The listing builds one solid part. Answer for the finished solid, in the listing's coordinates (mm). A direction names the side the tool comes from. Round coordinates to 2 decimals unless told otherwise and drop trailing zeros. Write each loop counter-clockwise with the first axis right and the second up, starting at its lowest first coordinate (ties: lowest second). Pieces come first, ordered by that corner, then holes. Notation, with made-up numbers: M -39,-12 L -7,-12 A33 cw -7,19 Z; hole C 71.5,87 d7. An arc over 180 degrees is marked long. Write each question's results on one line, items separated by ' | '.
from build123d import *

# Parameters (mm, degrees)
SKETCH_1_R          = 42.5
EXTRUDE_1_DEPTH     = 5
SKETCH_2_R          = 5.15
CUT_EXTRUDE_1_DEPTH = 61.311690409
SKETCH_3_R          = 5.15
CUT_EXTRUDE_2_DEPTH = 61.311690409
EXTRUDE_START       = -1
SKETCH_4_R          = 5.15
SKETCH_4_R_2        = 4.15
EXTRUDE_1_2_DEPTH   = 1
CUT_EXTRUDE_3_REACH = 62.312
SKETCH_5_R          = 1.65
CUT_EXTRUDE_4_REACH = 62.312
CUT_EXTRUDE_6_REACH = 62.312
SKETCH_10_R         = 2.15
CUT_EXTRUDE_7_REACH = 62.312
SKETCH_17_W         = 15.112394154
SKETCH_17_H         = 1
EXTRUDE_6_DEPTH     = 5


with BuildPart() as part:
    # 草图1 → Extrude 1 (new body)
    with BuildSketch(Plane.XY):
        Circle(SKETCH_1_R)
    extrude(amount=-EXTRUDE_1_DEPTH)

    # 草图2 → 切除-拉伸1 (cut, through all)
    with BuildSketch(Plane.XY):
        with Locations((-32, 0)):
            Circle(SKETCH_2_R)
        with Locations((-16, 27.712812921)):
            Circle(SKETCH_2_R)
        with Locations((16, 27.712812921)):
            Circle(SKETCH_2_R)
        with Locations((32, 0)):
            Circle(SKETCH_2_R)
        with Locations((16, -27.712812921)):
            Circle(SKETCH_2_R)
        with Locations((-16, -27.712812921)):
            Circle(SKETCH_2_R)
    extrude(amount=-CUT_EXTRUDE_1_DEPTH, mode=Mode.SUBTRACT)

    # 草图3 → 切除-拉伸2 (cut, through all)
    with BuildSketch(Plane.XY):
        Circle(SKETCH_3_R)
    extrude(amount=-CUT_EXTRUDE_2_DEPTH, mode=Mode.SUBTRACT)

    # 草图4 → Extrude 1 2 (add)
    # profile 1 of 6: a face of its own
    with BuildSketch(Plane(origin=(0, 0, -5), x_dir=(-1, 0, 0), z_dir=(0, 0, -1)).offset(EXTRUDE_START)):
        with Locations((-16, 27.712812921)):
            Circle(SKETCH_4_R)
        with Locations((-16, 27.712812921)):
            Circle(SKETCH_4_R_2, mode=Mode.SUBTRACT)
    # profile 2 of 6: a face of its own
    with BuildSketch(Plane(origin=(0, 0, -5), x_dir=(-1, 0, 0), z_dir=(0, 0, -1)).offset(EXTRUDE_START)):
        with Locations((16, 27.712812921)):
            Circle(SKETCH_4_R)
        with Locations((16, 27.712812921)):
            Circle(SKETCH_4_R_2, mode=Mode.SUBTRACT)
    # profile 3 of 6: a face of its own
    with BuildSketch(Plane(origin=(0, 0, -5), x_dir=(-1, 0, 0), z_dir=(0, 0, -1)).offset(EXTRUDE_START)):
        with Locations((32, 0)):
            Circle(SKETCH_4_R)
        with Locations((32, 0)):
            Circle(SKETCH_4_R_2, mode=Mode.SUBTRACT)
    # profile 4 of 6: a face of its own
    with BuildSketch(Plane(origin=(0, 0, -5), x_dir=(-1, 0, 0), z_dir=(0, 0, -1)).offset(EXTRUDE_START)):
        with Locations((16, -27.712812921)):
            Circle(SKETCH_4_R)
        with Locations((16, -27.712812921)):
            Circle(SKETCH_4_R_2, mode=Mode.SUBTRACT)
    # profile 5 of 6: a face of its own
    with BuildSketch(Plane(origin=(0, 0, -5), x_dir=(-1, 0, 0), z_dir=(0, 0, -1)).offset(EXTRUDE_START)):
        with Locations((-16, -27.712812921)):
            Circle(SKETCH_4_R)
        with Locations((-16, -27.712812921)):
            Circle(SKETCH_4_R_2, mode=Mode.SUBTRACT)
    # profile 6 of 6: a face of its own
    with BuildSketch(Plane(origin=(0, 0, -5), x_dir=(-1, 0, 0), z_dir=(0, 0, -1)).offset(EXTRUDE_START)):
        with Locations((-32, 0)):
            Circle(SKETCH_4_R)
        with Locations((-32, 0)):
            Circle(SKETCH_4_R_2, mode=Mode.SUBTRACT)
    extrude(amount=EXTRUDE_1_2_DEPTH)

    # 草图5 → 切除-拉伸3 (cut, up to next)
    with BuildSketch(Plane(origin=(0, 0, -5), x_dir=(-1, 0, 0), z_dir=(0, 0, -1)), mode=Mode.PRIVATE) as cut_extrude_3_sk1:
        with Locations((-16.454482672, 9.5)):
            Circle(SKETCH_5_R)
    cut_extrude_3_tool1 = extrude(cut_extrude_3_sk1.sketch, amount=-CUT_EXTRUDE_3_REACH, mode=Mode.PRIVATE) & part.part
    # 草图5 → 切除-拉伸3 (cut, up to next)
    with BuildSketch(Plane(origin=(0, 0, -5), x_dir=(-1, 0, 0), z_dir=(0, 0, -1)), mode=Mode.PRIVATE) as cut_extrude_3_sk2:
        with Locations((16.454482672, 9.5)):
            Circle(SKETCH_5_R)
    cut_extrude_3_tool2 = extrude(cut_extrude_3_sk2.sketch, amount=-CUT_EXTRUDE_3_REACH, mode=Mode.PRIVATE) & part.part
    # 草图5 → 切除-拉伸3 (cut, up to next)
    with BuildSketch(Plane(origin=(0, 0, -5), x_dir=(-1, 0, 0), z_dir=(0, 0, -1)), mode=Mode.PRIVATE) as cut_extrude_3_sk3:
        with Locations((0, -19)):
            Circle(SKETCH_5_R)
    cut_extrude_3_tool3 = extrude(cut_extrude_3_sk3.sketch, amount=-CUT_EXTRUDE_3_REACH, mode=Mode.PRIVATE) & part.part
    add(cut_extrude_3_tool1.solids().sort_by_distance((16.454483, 9.5, -5))[0], mode=Mode.SUBTRACT)
    add(cut_extrude_3_tool2.solids().sort_by_distance((-16.454483, 9.5, -5))[0], mode=Mode.SUBTRACT)
    add(cut_extrude_3_tool3.solids().sort_by_distance((0, -19, -5))[0], mode=Mode.SUBTRACT)

    # 草图7 → 切除-拉伸4 (cut, up to next)
    with BuildSketch(Plane(origin=(0, 0, -5), x_dir=(-1, 0, 0), z_dir=(0, 0, -1)), mode=Mode.PRIVATE) as cut_extrude_4_sk1:
        with BuildLine():
            Line((-16.495508076, -11.428941916), (-25.155762114, -16.428941916))
            ThreePointArc((-25.155762114, -16.428941916), (-27.40970403, -15.825), (-26.805762114, -13.571058084))
            Line((-26.805762114, -13.571058084), (-18.145508076, -8.571058084))
            ThreePointArc((-18.145508076, -8.571058084), (-15.891566159, -9.175), (-16.495508076, -11.428941916))
        make_face()
    cut_extrude_4_tool1 = extrude(cut_extrude_4_sk1.sketch, amount=-CUT_EXTRUDE_4_REACH, mode=Mode.PRIVATE) & part.part
    add(cut_extrude_4_tool1.solids().sort_by_distance((21.650635, -12.5, -5))[0], mode=Mode.SUBTRACT)

    # 草图10 → 切除-拉伸6 (cut, up to next)
    with BuildSketch(Plane(origin=(0, 0, -5), x_dir=(-1, 0, 0), z_dir=(0, 0, -1)), mode=Mode.PRIVATE) as cut_extrude_6_sk1:
        with Locations((-9.526279442, -5.5)):
            Circle(SKETCH_10_R)
    cut_extrude_6_tool1 = extrude(cut_extrude_6_sk1.sketch, amount=-CUT_EXTRUDE_6_REACH, mode=Mode.PRIVATE) & part.part
    # 草图10 → 切除-拉伸6 (cut, up to next)
    with BuildSketch(Plane(origin=(0, 0, -5), x_dir=(-1, 0, 0), z_dir=(0, 0, -1)), mode=Mode.PRIVATE) as cut_extrude_6_sk2:
        with Locations((0, 11)):
            Circle(SKETCH_10_R)
    cut_extrude_6_tool2 = extrude(cut_extrude_6_sk2.sketch, amount=-CUT_EXTRUDE_6_REACH, mode=Mode.PRIVATE) & part.part
    # 草图10 → 切除-拉伸6 (cut, up to next)
    with BuildSketch(Plane(origin=(0, 0, -5), x_dir=(-1, 0, 0), z_dir=(0, 0, -1)), mode=Mode.PRIVATE) as cut_extrude_6_sk3:
        with Locations((9.526279442, -5.5)):
            Circle(SKETCH_10_R)
    cut_extrude_6_tool3 = extrude(cut_extrude_6_sk3.sketch, amount=-CUT_EXTRUDE_6_REACH, mode=Mode.PRIVATE) & part.part
    add(cut_extrude_6_tool1.solids().sort_by_distance((9.526279, -5.5, -5))[0], mode=Mode.SUBTRACT)
    add(cut_extrude_6_tool2.solids().sort_by_distance((0, 11, -5))[0], mode=Mode.SUBTRACT)
    add(cut_extrude_6_tool3.solids().sort_by_distance((-9.526279, -5.5, -5))[0], mode=Mode.SUBTRACT)

    # 草图11 → 切除-拉伸7 (cut, up to next)
    with BuildSketch(Plane.XY, mode=Mode.PRIVATE) as cut_extrude_7_sk1:
        with BuildLine():
            Line((1.65, 25.457782029), (1.65, 18.457782029))
            ThreePointArc((1.65, 18.457782029), (0, 16.807782029), (-1.65, 18.457782029))
            Line((-1.65, 18.457782029), (-1.65, 25.457782029))
            ThreePointArc((-1.65, 25.457782029), (0, 27.107782029), (1.65, 25.457782029))
        make_face()
    cut_extrude_7_tool1 = extrude(cut_extrude_7_sk1.sketch, amount=-CUT_EXTRUDE_7_REACH, mode=Mode.PRIVATE) & part.part
    add(cut_extrude_7_tool1.solids().sort_by_distance((0, 21.957782, 0))[0], mode=Mode.SUBTRACT)

    # 草图17 → 拉伸-薄壁6 (add)
    with BuildSketch(Plane(origin=(0, 0, -5), x_dir=(-1, 0, 0), z_dir=(0, 0, -1))):
        with Locations((0, 42)):
            Rectangle(SKETCH_17_W, SKETCH_17_H)
    extrude(amount=-EXTRUDE_6_DEPTH)


solid = part.part
1) Find the intervals of material crossed by line 1 (X direction, y = 2, z = -0.5); line 2 (Y direction, x = 18.5, z = -1.4); line 3 (Y direction, x = 16, z = -4.15), in increasing order.
Return value:
line 1: -42.45 to -36.75, -27.25 to -4.75, 4.75 to 27.25, 36.75 to 42.45 | line 2: -38.26 to -32.22, -23.21 to -12.59, -8.78 to 23.21, 32.22 to 38.26 | line 3: -39.37 to -31.86, -23.56 to -10.99, -9.01 to 7.91, 11.09 to 23.56, 31.86 to 39.37
2) The mould has two halves that part along X. Classify faces 3 (the face through (0, 42.5, -3)), 4 (the face through (-1.762, -42.463, -2.465)), 5 (the face through (-12.71, -30.24, -4.49)): +X half, -X half, draft (parallel to the pull), parting line (faces both ways), or undercut.
Return value:
face 3: draft | face 4: parting line | face 5: undercut
3) Section D-D (x = -32) is taken. Determine the outline of the cut face in (y, z), then the cut area to 3 significant figures.
Return value:
outline: M -27.97,-5 L -4.15,-5 L -4.15,-4 L -5.15,-4 L -5.15,0 L -27.97,0 Z; M 4.15,-5 L 27.97,-5 L 27.97,0 L 5.15,0 L 5.15,-4 L 4.15,-4 Z | area: 230 mm²
4) A tool of negligible diameter and unlimited length cuts with its end or side. For faces 1 (the face through (20.765, -13.894, -2.535)), 2 (the face through (-37.145, 0.226, -1.972)), from which of +Z, -Z, +X, -X, +Y, -Y can it reach the whole face along a straight path? Write none if from no direction.
Return value:
face 1: +Z, -Z | face 2: +Z
5) Section B-B (y = -6.5) is taken. Determine the outline of the cut face in (x, z), then the cut area to 3 significant figures.
Return value:
outline: M -42,-5 L -11.43,-5 L -11.43,0 L -42,0 Z; M -7.62,-5 L 7.62,-5 L 7.62,0 L -7.62,0 Z; M 11.43,-5 L 42,-5 L 42,0 L 11.43,0 Z | area: 382 mm²
6) Section C-C (y = -15) is taken. Determine the outline of the cut face in (x, z).
Return value:
outline: M -39.76,-5 L 22.68,-5 L 22.68,0 L -39.76,0 Z; M 27.63,-5 L 39.76,-5 L 39.76,0 L 27.63,0 Z
7) Section A-A (x = 0) is taken. Determine the outline of the cut face in (y, z).
Return value:
outline: M -42.5,-5 L -20.65,-5 L -20.65,0 L -42.5,0 Z; M -17.35,-5 L -5.15,-5 L -5.15,0 L -17.35,0 Z; M 5.15,-5 L 8.85,-5 L 8.85,0 L 5.15,0 Z; M 13.15,-5 L 16.81,-5 L 16.81,0 L 13.15,0 Z; M 27.11,-5 L 42.5,-5 L 42.5,0 L 27.11,0 Z
8) Each of these flat-tipped pins is pushed along its axis until it touches: pin 1 (1 mm diameter, centred on x = 26.5, y = 33.5, fed in from +Z); pin 2 (2 mm diameter, centred on y = -19.5, z = -4.5, fed in from +X). Where does it stop, or does it pass through?
Return value:
pin 1: z = 0 | pin 2: x = 38.26
